For this review, take the finished solid that the model builds, in its own axes (mm). A direction names the side the tool comes from. Round coordinates to 2 decimals unless told otherwise and drop trailing zeros. Write each loop counter-clockwise with the first axis right and the second up, starting at its lowest first coordinate (ties: lowest second). Pieces come first, ordered by that corner, then holes. Notation, with made-up numbers: M 54,59.5 L 83,59.5 A13 ccw 83,63.5 Z; hole C 76,9.25 d8. An arc over 180 degrees is marked long. Answer in a Markdown table with one row per item.
Autodesk Inventor part; units mm, degrees
ref_plane "YZ Plane" through (0, 0, 0) normal (1, 0, 0) x (0, 1, 0)
ref_plane "XZ Plane" through (0, 0, 0) normal (0, 1, 0) x (-1, 0, 0)
ref_plane "XY Plane" through (0, 0, 0) normal (0, 0, 1) x (1, 0, 0)
sketch "Sketch1" plane through (0, 0, 0) normal (1, 0, 0) x (0, 1, 0)
  line L0 (4.3954, 24.8951) -> (-24.8146, 24.8951)
  line L1 (-30.2756, 19.4341) -> (-30.2756, -19.8089)
  line L2 (-24.8146, -25.2699) -> (4.3954, -25.2699)
  line L3 (9.8564, -19.8089) -> (9.8564, 19.4341)
  arc A0 (4.3954, -25.2699) -> (9.8564, -19.8089) centre (4.3954, -19.8089) ccw
  arc A1 (9.8564, 19.4341) -> (4.3954, 24.8951) centre (4.3954, 19.4341) ccw
  arc A2 (-30.2756, -19.8089) -> (-24.8146, -25.2699) centre (-24.8146, -19.8089) ccw
  arc A3 (-24.8146, 24.8951) -> (-30.2756, 19.4341) centre (-24.8146, 19.4341) ccw
  point P0 (0, 0)
  point P1 (-30.2756, -25.2699)
  point P2 (-30.2756, 24.8951)
  point P3 (9.8564, -25.2699)
  dimension "d0" = 40.132
  dimension "d1" = 50.165
  dimension "d2" = 5.461
  dimension "d3" = 5.461
extrude "Extrusion1" add sketch "Sketch1" along normal blind 7.62
sketch "Sketch2" plane through (0, 0, 0) normal (-1, 0, 0) x (0, 0, 1)
  line L0 (-25.2699, -24.8146) -> (-25.2699, 4.3954)
  line L1 (-25.2699, 4.3954) -> (-20.1899, 4.3954)
  line L2 (-20.1899, 4.3954) -> (-20.1899, 9.8564)
  line L3 (19.4341, 9.8564) -> (-19.8089, 9.8564)
  line L4 (-20.1899, 7.1259) -> (-5.4579, 7.1259)
  line L5 (-5.4579, 7.1259) -> (-5.4579, -7.6061)
  line L6 (-5.4579, -7.6061) -> (-20.1899, -7.6061)
  line L7 (-20.1899, -7.6061) -> (-20.1899, 7.1259)
  circle A0 centre (-12.8239, -0.2401) radius 7.366
  point P0 (0, 0)
  dimension "d6" = 5.08
  dimension "d7" = 14.732
  dimension "d8" = 14.732
  dimension "d9" = 14.732
extrude "Extrusion2" cut sketch "Sketch2" against normal up to next contours A0
sketch "Sketch3" plane through (0, 0, 0) normal (-1, 0, 0) x (0, 0, 1)
  point P0 (0, 0)
sketch "Sketch4" plane through (0, 0, 0) normal (-1, 0, 0) x (0, 0, 1)
  arc A0 (24.8951, 4.3954) -> (19.4341, 9.8564) centre (19.8306, 4.7919) ccw
  line L0 (19.4341, 9.8564) -> (19.4341, 8.5864)
  line L1 (19.4341, 8.5864) -> (4.7021, 8.5864)
  line L2 (4.7021, 8.5864) -> (4.7021, -6.1456)
  line L3 (4.7021, -6.1456) -> (19.4341, -6.1456)
  line L4 (19.4341, -6.1456) -> (19.4341, 8.5864)
  point P0 (0, 0)
  dimension "d13" = 1.27
  dimension "d14" = 14.732
  dimension "d15" = 14.732
extrude "Extrusion3" cut sketch "Sketch4" against normal up to next
sketch "Sketch5" plane through (0, 0, 0) normal (-1, 0, 0) x (0, 0, 1)
  line L0 (20.1796, -20.03) -> (6.1455, -28.1326)
  line L1 (6.1455, -28.1326) -> (6.1455, -11.9274)
  line L2 (6.1455, -11.9274) -> (20.1796, -20.03)
  line L3 (4.3902, -29.2503) -> (21.3615, -29.2503)
  point P0 (0, 0)
  point P1 (10.8235, -20.03)
  dimension "d18" = 16.2052
extrude "Extrusion4" cut sketch "Sketch5" against normal up to next
sketch "Sketch6" plane through (0, 0, 0) normal (-1, 0, 0) x (0, 0, 1)
  line L0 (19.4341, -30.2756) -> (-19.8089, -30.2756)
  line L1 (-24.8889, -30.2756) -> (-19.8089, -30.2756)
  line L2 (-19.8089, -30.2756) -> (-19.8089, -29.0056)
  line L3 (-19.8089, -29.0056) -> (-5.0769, -29.0056) construction
  line L4 (-5.0769, -29.0056) -> (-5.0769, -14.2736)
  line L5 (-5.0769, -14.2736) -> (-19.8089, -14.2736) construction
  line L6 (-19.8089, -14.2736) -> (-19.8089, -29.0056) construction
  circle A0 centre (-12.47, -21.7171) radius 7.4436 construction
  line L7 (-8.0948, -15.6951) -> (-5.3908, -24.0173) construction
  line L8 (-5.3908, -24.0173) -> (-12.47, -29.1607) construction
  line L9 (-12.47, -29.1607) -> (-19.5493, -24.0173) construction
  line L10 (-19.5493, -24.0173) -> (-16.8452, -15.6951) construction
  line L11 (-16.8452, -15.6951) -> (-8.0948, -15.6951) construction
  line L12 (-12.47, -21.7171) -> (-5.3908, -24.0173) construction
  line L13 (-12.47, -21.7171) -> (-8.0948, -15.6951) construction
  line L14 (-12.47, -21.7171) -> (-16.8452, -15.6951) construction
  line L15 (-12.47, -21.7171) -> (-19.5493, -24.0173) construction
  line L16 (-16.8452, -15.6951) -> (-11.847, -15.6951) construction
  line L17 (-12.47, -29.1607) -> (-7.7202, -29.1607) construction
  line L18 (-12.47, -21.7171) -> (-12.47, -29.1607) construction
  line L19 (-12.47, -21.7171) -> (-6.7428, -19.8562) construction
  line L20 (-8.0948, -15.6951) -> (-7.9391, -20.2449)
  line L21 (-7.9391, -20.2449) -> (-5.3908, -24.0173)
  line L22 (-12.47, -21.7171) -> (-8.9304, -26.589) construction
  line L23 (-5.3908, -24.0173) -> (-9.9432, -25.195)
  line L24 (-12.47, -29.1607) -> (-9.9432, -25.195)
  line L25 (-12.47, -21.7171) -> (-16.0096, -26.589) construction
  line L26 (-12.47, -21.7171) -> (-18.666, -19.7714) construction
  line L27 (-12.47, -21.7171) -> (-12.4334, -15.6951) construction
  line L28 (-19.5493, -24.0173) -> (-16.8734, -20.3343)
  line L29 (-16.8452, -15.6951) -> (-16.8734, -20.3343)
  line L30 (-16.8452, -15.6951) -> (-12.4404, -16.8346)
  line L31 (-12.4404, -16.8346) -> (-8.0948, -15.6951)
  line L32 (-19.5493, -24.0173) -> (-14.9968, -25.195)
  line L33 (-14.9968, -25.195) -> (-12.47, -29.1607)
  point P0 (0, 0)
  point P1 (-12.2672, -15.6951)
  dimension "d21" = 5.08
  dimension "d22" = 1.27
  dimension "d23" = 14.732
  dimension "d24" = 14.732
  dimension "d33" = 4.5524
  dimension "d34" = 4.5524
sketch "Sketch7" plane through (0, 0, 0) normal (-1, 0, 0) x (0, 0, 1)
  point P0 (0, 0)
sketch "Sketch8" plane through (0, 0, 0) normal (-1, 0, 0) x (0, 0, 1)
  point P0 (0, 0)
sketch "Sketch9" plane through (0, 0, 0) normal (-1, 0, 0) x (0, 0, 1)
  point P0 (0, 0)
extrude "Extrusion5" cut sketch "Sketch6" against normal up to next
properties part number "Passenger base"
Q1. Take a section at D-D (y = -12.5). State the section outline as (x, z) points.
Found:
| item | result |
|---|---|
| outline | M 0,-25.27 L 7.62,-25.27 L 7.62,6.15 L 0,6.15 Z; M 0,7.14 L 7.62,7.14 L 7.62,24.9 L 0,24.9 Z |
Q2. For probe 1 along Y at (x, z) = (4.75, 5); probe 2 along Z at (x, y) = (3.5, -2.5); probe 3 along Z at (x, y) = (2.25, 0), list the stretches that pass through material, from the lowest coordinate up.
Found:
| item | result |
|---|---|
| probe 1 | -30.28 to -6.15, 8.59 to 9.86 |
| probe 2 | -25.27 to -19.83, -5.81 to 4.7, 19.43 to 24.9 |
| probe 3 | -25.27 to -20.19, -5.46 to 4.7, 19.43 to 24.9 |
Q3. Take a section at C-C (x = 6). State the section outline as (y, z) points (1 decimal), then the cut area to 3 significant figures.
Found:
| item | result |
|---|---|
| outline | M -30.3,-19.8 A5.5 ccw -24.8,-25.3 L 4.4,-25.3 A5.5 ccw 9.9,-19.8 L 9.9,19.4 A5.5 ccw 4.4,24.9 L -24.8,24.9 A5.5 ccw -30.3,19.4 Z; hole M -29.2,-12.5 L -25.2,-15 L -24,-19.5 L -20.3,-16.9 L -15.7,-16.8 L -16.8,-12.4 L -15.7,-8.1 L -20.2,-7.9 L -24,-5.4 L -25.2,-9.9 Z; hole M -28.1,6.1 L -11.9,6.1 L -20,20.2 Z; hole C -0.2,-12.8 d14.7; hole M -6.1,4.7 L 8.6,4.7 L 8.6,19.4 L -6.1,19.4 Z |
| area | 1,390 mm² |
Q4. Machinability: for faces 1 (the face through (4, -10, -25.27)), 2 (the face through (3.76, -22.2, -18.23)), which of the approach directions +Z, -Z, +X, -X, +Y, -Y give a long, thin tool a straight path to every point of the face, cutting with its end or side? Answer none if there is none.
Found:
| item | result |
|---|---|
| face 1 | -Z, +X, -X, +Y, -Y |
| face 2 | +X, -X |
Q5. Take a section at B-B (y = -26). State the section outline as (x, z) points, then the cut area to 3 significant figures.
Found:
| item | result |
|---|---|
| outline | M 0,-25.14 L 7.62,-25.14 L 7.62,-14.48 L 0,-14.48 Z; M 0,-10.46 L 7.62,-10.46 L 7.62,6.15 L 0,6.15 Z; M 0,9.84 L 7.62,9.84 L 7.62,24.76 L 0,24.76 Z |
| area | 321 mm² |
Q6. Take a section at A-A (z = -17.5). State the section outline as (x, y) points, then the cut area to 3 significant figures.
Found:
| item | result |
|---|---|
| outline | M 0,-30.28 L 7.62,-30.28 L 7.62,-24.55 L 0,-24.55 Z; M 0,-21.2 L 7.62,-21.2 L 7.62,-5.93 L 0,-5.93 Z; M 0,5.45 L 7.62,5.45 L 7.62,9.86 L 0,9.86 Z |
| area | 194 mm² |
Q7. Mouldability with a two-part tool opening along Y and no side actions: class faces 3 (the face through (4, 8.586, 12)), 4 (the face through (3.757, 8.299, -23.628)), 5 (the face through (3.757, -28.633, -23.713)), 6 (the face through (4, -20, 6.146)) as +Y half, -Y half, draft (parallel to the pull), parting line (faces both ways), or undercut.
Found:
| item | result |
|---|---|
| face 3 | undercut |
| face 4 | +Y half |
| face 5 | -Y half |
| face 6 | undercut |
